Could you check a few things on this model? Use its own coordinates, in mm. Coordinates: 2 decimals unless noted, no trailing zeros. Write each loop counter-clockwise with the first axis right and the second up, starting at its lowest first coordinate (ties: lowest second). Pieces come first, ordered by that corner, then holes.
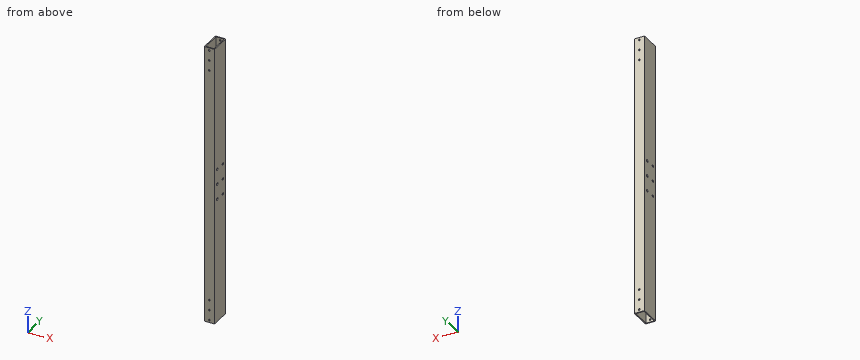
```python
from build123d import *

# Parameters (mm, degrees)
SKETCH1_W           = 25.4
SKETCH1_H           = 50.8
SKETCH1_W_2         = 20.32
SKETCH1_H_2         = 45.72
EXTRUDE_THIN1_DEPTH = 698.5
SKETCH2_R           = 2.0701
CUT_EXTRUDE1_DEPTH  = 701.459977443
SKETCH3_R           = 3.175
CUT_EXTRUDE2_DEPTH  = 700.423026501


with BuildPart() as part:
    # Sketch1 → Extrude-Thin1 (new body)
    with BuildSketch(Plane.XY):
        Rectangle(SKETCH1_W, SKETCH1_H)
        Rectangle(SKETCH1_W_2, SKETCH1_H_2, mode=Mode.SUBTRACT)
    extrude(amount=EXTRUDE_THIN1_DEPTH)

    # Sketch2 → Cut-Extrude1 (cut, through all)
    with BuildSketch(Plane(origin=(0, 25.4, 0), x_dir=(1, 0, 0), z_dir=(0, 1, 0))):
        with Locations(Location((0, -6.35, 0), (0, 0, 270))):
            Circle(SKETCH2_R)
        with Locations(Location((0, -31.75, 0), (0, 0, 270))):
            Circle(SKETCH2_R)
        with Locations(Location((0, -57.15, 0), (0, 0, 270))):
            Circle(SKETCH2_R)
        with Locations(Location((0, -641.35, 0), (0, 0, 270))):
            Circle(SKETCH2_R)
        with Locations(Location((0, -666.75, 0), (0, 0, 270))):
            Circle(SKETCH2_R)
        with Locations(Location((0, -692.15, 0), (0, 0, 270))):
            Circle(SKETCH2_R)
    extrude(amount=-CUT_EXTRUDE1_DEPTH, mode=Mode.SUBTRACT)

    # Sketch3 → Cut-Extrude2 (cut, through all)
    with BuildSketch(Plane.ZY.offset(12.7)):
        with Locations((311.15, 12.7)):
            Circle(SKETCH3_R)
        with Locations((311.15, -12.7)):
            Circle(SKETCH3_R)
        with Locations((387.35, -12.7)):
            Circle(SKETCH3_R)
        with Locations((387.35, 12.7)):
            Circle(SKETCH3_R)
        with Locations((349.25, 12.7)):
            Circle(SKETCH3_R)
        with Locations((349.25, -12.7)):
            Circle(SKETCH3_R)
    extrude(amount=-CUT_EXTRUDE2_DEPTH, mode=Mode.SUBTRACT)


solid = part.part
```
1. I want a section at A-A on z = 147.5. Please give me the cut outline in (x, y).
Verdict:
outline: (-12.7, -25.4) - (12.7, -25.4) - (12.7, 25.4) - (-12.7, 25.4) - close; hole (-10.16, -22.86) - (10.16, -22.86) - (10.16, 22.86) - (-10.16, 22.86) - close
2. For pin 1 (2.5 mm diameter, centred on x = 0, z = 31.75, fed in from -Y), with a flat end and sliding along its axis, tell me the tip position at first contact or that it passes through.
Verdict:
pin 1: passes through
3. Please list where these lines run through material, in increasing order: line 1 along Y through (x, z) = (11.3, 349.25) (3 decimals); line 2 along Y through (x, z) = (5.25, 359.5); line 3 along X through (y, z) = (-1, 364.5).
Verdict:
line 1: y = -25.4 to -15.875, -9.525 to 9.525, 15.875 to 25.4
line 2: y = -25.4 to -22.86, 22.86 to 25.4
line 3: x = -12.7 to -10.16, 10.16 to 12.7
